from build123d import *

# Parameters (mm, degrees)
F0_R     = 23.01875
F0_R_2   = 3.96875
F0_R_3   = 2.15265
F0_R_4   = 11.90625
F1_DEPTH = 3.175


with BuildPart() as f1:
    # F0 (on Top) → F1 (new body)
    with BuildSketch(Plane.XY):
        Circle(F0_R)
        with Locations((-12.347852, -12.347852)):
            Circle(F0_R_2, mode=Mode.SUBTRACT)
        with Locations((12.347852, -12.347852)):
            Circle(F0_R_3, mode=Mode.SUBTRACT)
        with Locations((-12.347852, 12.347852)):
            Circle(F0_R_3, mode=Mode.SUBTRACT)
        Circle(F0_R_4, mode=Mode.SUBTRACT)
        with Locations((12.347852, 12.347852)):
            Circle(F0_R_2, mode=Mode.SUBTRACT)
    extrude(amount=F1_DEPTH)


solid = f1.part
Source: CAD feature listing. Evaluate the final solid. Frame: model axes, mm. Round coordinates to 2 decimals unless told otherwise and drop trailing zeros. Loops run counter-clockwise (first coordinate to the right, second up) from the corner with the lowest first, then second, coordinate; pieces in that order, holes last. Notation, with made-up numbers: (-39.5, 47.25) - (-28.5, 47.25) arc R23 ccw to (-28.5, 78.25) - close; hole circle Ø3 at (-7.5, 66). An arc over 180 degrees is marked (long way). Write item = value, one per line. Start each with the question number.
(1) Section query A-A, the plane x = 0. Output: boundary loops of the cut face in (y, z) (3 decimals).
(2) Pin query (flat end, axial travel): pin 1 (1 mm diameter, centred on x = -1.5, z = 3, fed in from -Y). Return the tip coordinate at first contact, or that it passes through.
(3) Ray query, line 1 along Y through (x, z) = (-10, 0.3); line 2 along X through (y, z) = (-12, 2.5); line 3 along Y through (x, z) = (-9.5, 0.45). Return the intervals inside material, ascending. Write a range as from..to.
(4) Section query C-C, the plane z = 1.85. Output: boundary loops of the cut face in (x, y).
(5) Pull-direction query (Y, two-part tool) for faces 1 (the face through (-9.45, -7.24, 1.57)), 2 (the face through (10, -10, 0)), 3 (the face through (-18.267, -14.007, 1.565)); classes: +Y half, -Y half, draft (parallel to the pull), parting line (faces both ways), or undercut.
Conclusion:
q1.outline = (-23.019, 0) - (-11.906, 0) - (-11.906, 3.175) - (-23.019, 3.175) - close; (11.906, 0) - (23.019, 0) - (23.019, 3.175) - (11.906, 3.175) - close
q2.pin_1 = -23
q3.line_1 = -20.73..-15.55, -9.15..-6.46, 6.46..20.73
q3.line_2 = -19.64..-16.3, -8.39..10.22, 14.47..19.64
q3.line_3 = -20.97..-15.11, -9.58..-7.18, 7.18..20.97
q4.outline = circle Ø46.04 at (0, 0); hole circle Ø7.94 at (-12.35, -12.35); hole circle Ø4.31 at (-12.35, 12.35); hole circle Ø23.81 at (0, 0); hole circle Ø7.94 at (12.35, 12.35); hole circle Ø4.31 at (12.35, -12.35)
q5.face_1 = undercut
q5.face_2 = draft
q5.face_3 = parting line
